Could you check a few things on this model? Use its own coordinates, in mm. A direction names the side the tool comes from. Coordinates: 2 decimals unless noted, no trailing zeros. Loops run counter-clockwise (first coordinate to the right, second up) from the corner with the lowest first, then second, coordinate; pieces in that order, holes last. Notation, with made-up numbers: (-6, 62.5) -> (30, 62.5) arc R18 ccw to (30, 84.5) -> close; hole circle Ø10 at (49, 45.25). An arc over 180 degrees is marked (long way). One line per question, with ' | ' between items.
from build123d import *

# Parameters (mm, degrees)
SKETCH_1_W          = 28.676374442
SKETCH_1_H          = 28.786423303
SKETCH_1_R          = 1
SKETCH_1_W_2        = 21.847787884
SKETCH_1_H_2        = 21.847787883
EXTRUDE_1_DEPTH     = 3
FILLET_1_R          = 2
SKETCH_2_R          = 12.563691981
EXTRUDE_2_DEPTH     = 5.5
SKETCH_3_W          = 30.61596727
SKETCH_3_H          = 31.734673245
SKETCH_3_R          = 1
SKETCH_3_W_2        = 23.133890408
SKETCH_3_H_2        = 23.048584014
EXTRUDE_3_DEPTH     = 1
SKETCH_5_R          = 10.591689203
SKETCH_5_R_2        = 8.299790342
CUT_EXTRUDE_1_DEPTH = 1.5
FILLET_2_R          = 3


with BuildPart() as part:
    # 草图1 → 凸台-拉伸1 (new body)
    with BuildSketch(Plane.XY):
        with Locations((4.252772695, -4.754098361)):
            Rectangle(SKETCH_1_W, SKETCH_1_H)
        with Locations((-8.247227305, 7.745901639)):
            Circle(SKETCH_1_R, mode=Mode.SUBTRACT)
        with Locations((16.752772695, 7.745901639)):
            Circle(SKETCH_1_R, mode=Mode.SUBTRACT)
        with Locations((16.752772695, -17.254098361)):
            Circle(SKETCH_1_R, mode=Mode.SUBTRACT)
        with Locations((-8.247227305, -17.254098361)):
            Circle(SKETCH_1_R, mode=Mode.SUBTRACT)
        with Locations((4.252772695, -4.754098361)):
            Rectangle(SKETCH_1_W_2, SKETCH_1_H_2, mode=Mode.SUBTRACT)
    extrude(amount=EXTRUDE_1_DEPTH)

    # 圆角1
    fillet_1_edges = [part.edges().sort_by_distance(p)[0] for p in [
        (18.590959916, -19.147310012, 1.5),
        (-10.085414526, -19.147310012, 1.5),
        (-10.085414526, 9.639113291, 1.5),
        (18.590959916, 9.639113291, 1.5),
    ]]
    fillet(fillet_1_edges, radius=FILLET_1_R)

    # 草图2 → 凸台-拉伸2 (add, symmetric)
    with BuildSketch(Plane.XY.offset(3)):
        with Locations((4.123944992, -4.882926064)):
            Circle(SKETCH_2_R)
    extrude(amount=EXTRUDE_2_DEPTH, both=True)

    # 草图3 → 凸台-拉伸3 (add)
    with BuildSketch(Plane.XY.offset(3)):
        with Locations((4.123944992, -4.882926064)):
            Rectangle(SKETCH_3_W, SKETCH_3_H)
        with Locations((-8.247227305, 7.745901639)):
            Circle(SKETCH_3_R, mode=Mode.SUBTRACT)
        with Locations((-8.247227305, -17.254098361)):
            Circle(SKETCH_3_R, mode=Mode.SUBTRACT)
        with Locations((16.752772695, -17.254098361)):
            Circle(SKETCH_3_R, mode=Mode.SUBTRACT)
        with Locations((16.752772695, 7.745901639)):
            Circle(SKETCH_3_R, mode=Mode.SUBTRACT)
        with Locations((4.123944992, -4.882926064)):
            Rectangle(SKETCH_3_W_2, SKETCH_3_H_2, mode=Mode.SUBTRACT)
    extrude(amount=EXTRUDE_3_DEPTH)

    # 草图5 → 切除-拉伸1 (cut)
    with BuildSketch(Plane.XY.offset(8.5)):
        with Locations((4.408371776, -4.882926064)):
            Circle(SKETCH_5_R)
        with Locations((4.408371776, -4.882926064)):
            Circle(SKETCH_5_R_2, mode=Mode.SUBTRACT)
    extrude(amount=-CUT_EXTRUDE_1_DEPTH, mode=Mode.SUBTRACT)

    # 圆角2
    fillet_2_edges = [part.edges().sort_by_distance(p)[0] for p in [
        (19.431928627, -20.750262686, 3.5),
        (19.431928627, 10.984410559, 3.5),
        (-11.184038643, 10.984410559, 3.5),
        (-11.184038643, -20.750262686, 3.5),
    ]]
    fillet(fillet_2_edges, radius=FILLET_2_R)


solid = part.part
1) If we section it at B-B on y = -15: Please give me the cut outline in (x, z), and give its area (3 significant figures).
Data:
outline: (-11.18, 3) -> (-10.09, 3) -> (-10.09, 0) -> (-6.67, 0) -> (-6.67, 3) -> (-7.44, 3) -> (-7.44, 4) -> (-11.18, 4) -> close; (-3.33, -2.5) -> (11.57, -2.5) -> (11.57, 8.5) -> (7.54, 8.5) -> (7.54, 7) -> (1.27, 7) -> (1.27, 8.5) -> (-3.33, 8.5) -> close; (15.18, 0) -> (18.59, 0) -> (18.59, 3) -> (19.43, 3) -> (19.43, 4) -> (15.69, 4) -> (15.69, 3) -> (15.18, 3) -> close | area: 182 mm²
2) If we section it at D-D on y = -3: Please give me the cut outline in (x, z).
Data:
outline: (-11.18, 3) -> (-10.09, 3) -> (-10.09, 0) -> (-8.3, 0) -> (-8.3, -2.5) -> (16.55, -2.5) -> (16.55, 0) -> (18.59, 0) -> (18.59, 3) -> (19.43, 3) -> (19.43, 4) -> (16.55, 4) -> (16.55, 8.5) -> (14.83, 8.5) -> (14.83, 7) -> (12.49, 7) -> (12.49, 8.5) -> (-3.68, 8.5) -> (-3.68, 7) -> (-6.01, 7) -> (-6.01, 8.5) -> (-8.3, 8.5) -> (-8.3, 4) -> (-11.18, 4) -> close
3) If we section it at A-A on x = 12: Please give me the cut outline in (y, z), and give its area (3 significant figures).
Data:
outline: (-20.75, 3) -> (-19.15, 3) -> (-19.15, 0) -> (-15.68, 0) -> (-15.68, 3) -> (-16.41, 3) -> (-16.41, 4) -> (-20.75, 4) -> close; (-14.67, -2.5) -> (4.91, -2.5) -> (4.91, 8.5) -> (2.5, 8.5) -> (2.5, 7) -> (-1.53, 7) -> (-1.53, 8.5) -> (-8.24, 8.5) -> (-8.24, 7) -> (-12.27, 7) -> (-12.27, 8.5) -> (-14.67, 8.5) -> close; (6.17, 0) -> (9.64, 0) -> (9.64, 3) -> (10.98, 3) -> (10.98, 4) -> (6.64, 4) -> (6.64, 3) -> (6.17, 3) -> close | area: 233 mm²
4) I'm going to push flat-ended pins straight in: pin 1 Ø1 at (x, z) = (11, 6.5) entering from -Y; pin 2 Ø2.5 at (y, z) = (-13.5, 2) entering from -X; pin 3 Ø3 at (x, y) = (16.75, 7.75) entering from +Z; pin 4 Ø2.5 at (y, z) = (-14, 1.5) entering from +X. Where does each tip first touch, or does it pass through?
Data:
pin 1: y = -15.71 | pin 2: x = -11.18 | pin 3: z = 4 | pin 4: x = 18.59
5) We'd pull the mould along Y, two halves only. Please class faces 1 (the face through (15.177, -13, 1)), 2 (the face through (4, -5, 8.5)), 3 (the face through (-10.33, 10.08, 3.51)): pulls with the +Y half, pulls with the -Y half, needs draft (parallel to the pull), parting line crosses it, or undercut.
Data:
face 1: undercut | face 2: needs draft | face 3: pulls with the +Y half
6) On a 3-axis mill with a long thin cutter (end or side, diameter ignored), from which of +Z, -Z, +X, -X, +Y, -Y can I reach the whole of each face in a straight line? I mean faces 4 (the face through (17.99, 9.07, 1.52)), 5 (the face through (-7.443, -13.1, 3.5)), 6 (the face through (13, 6.17, 1)). Say none if no direction works.
Data:
face 4: -Z, +X, +Y | face 5: +Z | face 6: +Z, -Z
7) If we section it at C-C on z = 1: Give the number of separate pieces and of enclosed holes in the cut face, and give its area (3 significant figures).
Data:
separate pieces: 1 | enclosed holes: 8 | area: 773 mm²
8) I need wall thicknesses on line 1 along X through (y, z) = (-13.5, 2); line 2 along Y through (x, z) = (-6, 1.5); line 3 along Z through (x, y) = (12.5, -17). Which ranges of each line are inside material? Lowest first, please. Write a range as from..to.
Data:
line 1: -10.09..-6.67, -5.02..13.27, 15.18..18.59 | line 2: -19.15..-15.68, -12.32..2.56, 6.17..9.64 | line 3: 0..4
